Autodesk Inventor part; units mm, degrees
ref_plane "YZ Plane" through (0, 0, 0) normal (1, 0, 0) x (0, 1, 0)
ref_plane "XZ Plane" through (0, 0, 0) normal (0, 1, 0) x (-1, 0, 0)
ref_plane "XY Plane" through (0, 0, 0) normal (0, 0, 1) x (1, 0, 0)
sketch "Náčrt1" plane through (0, 0, 0) normal (0, 0, 1) x (1, 0, 0)
  line L0 (-60, 10) -> (10, 10)
  line L1 (10, 10) -> (10, -10)
  line L2 (10, -10) -> (-60, -10)
  line L3 (-60, -10) -> (-60, 10)
  point P0 (0, 0)
  dimension "d0" = 20
  dimension "d1" = 70
  dimension "d2" = 10
  dimension "d3" = 10
extrude "Vysunutí1" add sketch "Náčrt1" along normal blind 0.5
sketch "Náčrt2" plane through (0, 0, 0.5) normal (0, 0, 1) x (1, 0, 0)
  circle A0 centre (-55, 5) radius 2
  line L0 (10, 10) -> (-60, 10)
  line L1 (-60, 10) -> (-60, -10)
  point P0 (0, 0)
  dimension "d6" = 4
  dimension "d7" = 5
  dimension "d8" = 5
extrude "Vysunutí2" cut sketch "Náčrt2" against normal blind 0.5
pattern_linear "Obdélníkové pole1" count 7 spacing 10 along (1, 0, 0) of "Vysunutí2"
fillet "Zaoblení1" radius 1 1 edges at (10, 10, 0.25)
fillet "Zaoblení2" radius 1 2 edges at (-60, 10, 0.25) (-60, -10, 0.25)
fillet "Zaoblení3" radius 1 1 edges at (10, -10, 0.25)
sketch "Náčrt3" plane through (0, 0, 0.5) normal (0, 0, 1) x (1, 0, 0)
  line L0 (7, -2.7639) -> (7, -7.2361)
  line L1 (3, -2.7639) -> (3, -7.2361)
  arc A0 (7, -2.7639) -> (3, -2.7639) centre (5, -5) ccw
  arc A1 (3, -7.2361) -> (7, -7.2361) centre (5, -5) ccw
  line L2 (10, -9) -> (10, 9)
  line L3 (-59, -10) -> (9, -10)
  point P0 (0, 0)
  point P1 (3, -7.229)
  point P2 (5, -8)
  point P3 (5, -2)
  dimension "d24" = 2
  dimension "d25" = 4
  dimension "d26" = 5
  dimension "d27" = 5
  dimension "d28" = 3
  dimension "d29" = 3
extrude "Vysunutí3" cut sketch "Náčrt3" against normal blind 10
pattern_linear "Obdélníkové pole2" count 7 spacing 10 along (-1, 0, 0) of "Vysunutí3"
properties part number "1021"
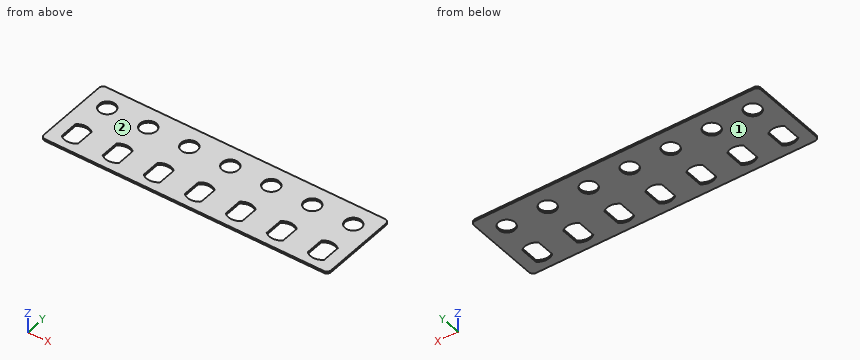
The model under review builds one solid part; all positions refer to its coordinate system, in mm. Face numbers are marked on the shaded views. Round coordinates to 2 decimals unless told otherwise and drop trailing zeros. Write each loop counter-clockwise with the first axis right and the second up, starting at its lowest first coordinate (ties: lowest second). Pieces come first, ordered by that corner, then holes.
(1) Mouldability with a two-part tool opening along Z and no side actions: class the marked faces 1 and 2 as +Z half, -Z half, draft (parallel to the pull), parting line (faces both ways), or undercut.
(2) We need section A-A on x = -5. Give the boundary of the cut face in (y, z), and give its area (3 significant figures).
(3) Wall thickness on L1, parallel to Y at x = -25, z = 0.15; L2, parallel to Y at x = -44.5, z = 0.35: over which ranges is each line inside the solid? List them lowest first.
(4) We need section B-B on y = 5. Give the number of separate pieces and of enclosed holes in the cut face, and give its area (3 significant figures).
Findings below:
1. face 1: -Z half
1. face 2: +Z half
2. outline: (-10, 0) - (-8, 0) - (-8, 0.5) - (-10, 0.5) - close; (-2, 0) - (3, 0) - (3, 0.5) - (-2, 0.5) - close; (7, 0) - (10, 0) - (10, 0.5) - (7, 0.5) - close
2. area: 5.00 mm2
3. L1: y = -10 to -8, -2 to 3, 7 to 10
3. L2: y = -10 to -7.96, -2.04 to 3.06, 6.94 to 10
4. separate pieces: 8
4. enclosed holes: 0
4. area: 21.0 mm2
